For this review, take the finished solid that the model builds, in its own axes (mm). Face numbers are marked on the shaded views. A direction names the side the tool comes from. Give positions to 0.01 mm unless a question says otherwise; leave off trailing zeros. Order: outer loops, then holes, each group sorted by start corner. A loop starts at its lowest first (then second) coordinate and runs counter-clockwise, first axis right, second up. Notation, with made-up numbers: (-10, -11) - (37, -11) arc R32 cw to (37, 21) - close; hole circle Ø11 at (59, 86). An arc over 180 degrees is marked (long way). Use a Markdown table: item, result. Add a question column.
1) We need section B-B on z = 56.5. Write out the cut boundary in (x, y).
2) Clearance check with flat-ended pins moving along their axes: P1, Ø4, axis at x = -2, z = 64.5, coming from the +Y side; P2, Ø2, axis at x = -7, z = 50, coming from the -Y side; P3, Ø10, axis at x = -8, z = 71, coming from the -Y side; P4, Ø6, axis at y = -15.5, z = 69, coming from the +X side. State where each tip first meets the part, or that it passes through.
3) Mouldability with a two-part tool opening along X and no side actions: class the marked faces 4, 5 and 6 as released by +X, released by -X, zero draft, split by the parting line, or undercut.
4) Wall thickness on L1, parallel to Y at x = -10.5, z = 71.5; L2, parallel to X at y = -3, z = 60.5; L3, parallel to Z at x = -31.5, y = 24.5: over which ranges is each line inside the solid? List them lowest first.
5) Machinability: for the marked faces 1, 2 and 3, which of the approach directions +Z, -Z, +X, -X, +Y, -Y give a long, thin tool a straight path to every point of the face, cutting with its end or side? Answer none if there is none.
6) We need section C-C on x = -7. Give the number of separate pieces and of enclosed holes in the cut face, then the cut area to 3 significant figures.
7) We need section D-D on y = -59. Write out the cut boundary in (x, z), then the cut area to 3 significant figures.
8) We need section A-A on y = 0. Write out the cut boundary in (x, z).
```python
from build123d import *

# Parameters (mm, degrees)
EXTRUDE_DEPTH           = 10
EXTRUDE_PLACEMENT_ANGLE = 90
CYLINDER004_R           = 38
CYLINDER004_DEPTH       = 30
CYLINDER003_R           = 4
CYLINDER003_DEPTH       = 140
CYLINDER005_R           = 20
CYLINDER005_DEPTH       = 10
CYLINDER_R              = 46
CYLINDER_DEPTH          = 60


with BuildPart() as extrude_body:
    # path2399 → Extrude (new body)
    with BuildSketch(Plane(origin=(8.682374, 337.01873, 81), x_dir=(0, 1, 0), z_dir=(0, 0, 1))):
        with BuildLine():
            add(Edge.make_bspline(
                [(-1.415579, 5.024931), (-1.938341, -2.484397)],
                knots=[0, 0, 7.527502, 7.527502], degree=1))
            add(Edge.make_bspline(
                [(-1.938341, -2.484397), (-1.938341, -2.484397), (-2.134903, -2.858259), (-2.273136, -3.334737)],
                knots=[0, 0, 0, 0, 1, 1, 1, 1], degree=3))
            add(Edge.make_bspline(
                [(-2.273136, -3.334737), (-2.411369, -3.811216), (-2.443203, -4.128926), (-2.371685, -4.540758)],
                knots=[0, 0, 0, 0, 1, 1, 1, 1], degree=3))
            add(Edge.make_bspline(
                [(-2.371685, -4.540758), (-2.300167, -4.952591), (-2.218933, -5.672599), (-1.772797, -6.040394)],
                knots=[0, 0, 0, 0, 1, 1, 1, 1], degree=3))
            add(Edge.make_bspline(
                [(-1.772797, -6.040394), (-1.326661, -6.40819), (-0.861351, -6.572675), (-0.583202, -6.662312)],
                knots=[0, 0, 0, 0, 1, 1, 1, 1], degree=3))
            add(Edge.make_bspline(
                [(-0.583202, -6.662312), (-0.305053, -6.751952), (0.507781, -6.731952), (0.709843, -6.630052)],
                knots=[0, 0, 0, 0, 1, 1, 1, 1], degree=3))
            add(Edge.make_bspline(
                [(0.709843, -6.630052), (0.911905, -6.52815), (1.481843, -6.245909), (1.726833, -5.892641)],
                knots=[0, 0, 0, 0, 1, 1, 1, 1], degree=3))
            add(Edge.make_bspline(
                [(1.726833, -5.892641), (1.971823, -5.539373), (2.340182, -5.059724), (2.384256, -4.759981)],
                knots=[0, 0, 0, 0, 1, 1, 1, 1], degree=3))
            add(Edge.make_bspline(
                [(2.384256, -4.759981), (2.42833, -4.460237), (2.223091, -3.691858), (2.158411, -3.465999)],
                knots=[0, 0, 0, 0, 1, 1, 1, 1], degree=3))
            add(Edge.make_bspline(
                [(2.158411, -3.465999), (2.093732, -3.240141), (1.863634, -2.929328), (1.863634, -2.929328)],
                knots=[0, 0, 0, 0, 1, 1, 1, 1], degree=3))
            add(Edge.make_bspline(
                [(1.863634, -2.929328), (1.423808, 5.709855)],
                knots=[0, 0, 8.650371, 8.650371], degree=1))
            add(Edge.make_bspline(
                [(1.423808, 5.709855), (1.423808, 5.709855), (1.246198, 6.226563), (0.794563, 6.495307)],
                knots=[0, 0, 0, 0, 1, 1, 1, 1], degree=3))
            add(Edge.make_bspline(
                [(0.794563, 6.495307), (0.342929, 6.764051), (-0.057622, 6.753041), (-0.37358, 6.666974)],
                knots=[0, 0, 0, 0, 1, 1, 1, 1], degree=3))
            add(Edge.make_bspline(
                [(-0.37358, 6.666974), (-0.689538, 6.580907), (-1.208145, 6.230265), (-1.306201, 5.897514)],
                knots=[0, 0, 0, 0, 1, 1, 1, 1], degree=3))
            add(Edge.make_bspline(
                [(-1.306201, 5.897514), (-1.404257, 5.564763), (-1.415579, 5.024931), (-1.415579, 5.024931)],
                knots=[0, 0, 0, 0, 1, 1, 1, 1], degree=3))
        make_face()
    extrude(amount=EXTRUDE_DEPTH)


with BuildPart() as extrude_body_1:
    # Extrude placement: moved
    add(extrude_body.part.moved(Location((-13, -4, 402))).rotate(Axis((-13, -4, 402), (-1, 0, 0)), EXTRUDE_PLACEMENT_ANGLE))


with BuildPart() as cylinder004:
    # Cylinder004 → Cylinder004 (new body)
    with BuildSketch(Plane.XY.offset(56)):
        Circle(CYLINDER004_R)
    extrude(amount=CYLINDER004_DEPTH)


with BuildPart() as cut:
    # Cylinder003 → Cylinder003 (new body)
    with BuildSketch(Plane(origin=(0, 70, 65), x_dir=(1, 0, 0), z_dir=(0, -1, 0))):
        Circle(CYLINDER003_R)
    extrude(amount=CYLINDER003_DEPTH)

    # Cut: cut Cylinder004
    add(cylinder004.part, mode=Mode.SUBTRACT)


with BuildPart() as cut001:
    # Cylinder005 → Cylinder005 (new body)
    with BuildSketch(Plane(origin=(0, 80, 65), x_dir=(1, 0, 0), z_dir=(0, -1, 0))):
        Circle(CYLINDER005_R)
    extrude(amount=CYLINDER005_DEPTH)

    # Fusion: union Cut
    add(cut.part)

    # Cut001: cut Extrude body
    add(extrude_body_1.part, mode=Mode.SUBTRACT)


with BuildPart() as cylinder:
    # Cylinder → Cylinder (new body)
    with BuildSketch(Plane.XY):
        Circle(CYLINDER_R)
    extrude(amount=CYLINDER_DEPTH)


with BuildPart() as fusion001:
    # Sketch → Revolve (revolve)
    with BuildSketch(Plane.XZ):
        Polygon((0, 1), (34, 1), (38, 70), (42.057971, 70), (38, 0), (0, 0), align=None)
    revolve(axis=Axis((0, 0, 0), (0, 0, 1)))

    # Cut002: cut Cylinder
    add(cylinder.part, mode=Mode.SUBTRACT)

    # Fusion001: union Cut001
    add(cut001.part)


solid = fusion001.part
```
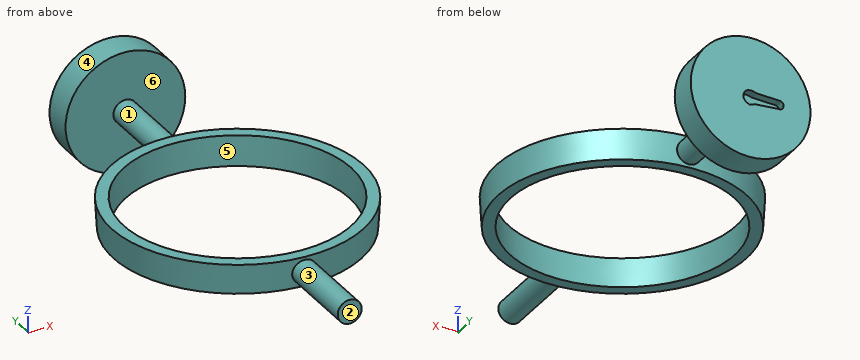
Checked values:
| question | item | result |
|---|---|---|
| 1 | outline | (-18.1, 70) - (18.1, 70) - (18.1, 80) - (-18.1, 80) - close |
| 2 | P1 | y = 80 |
| 2 | P2 | y = 70 |
| 2 | P3 | y = -41.94 |
| 2 | P4 | x = 40.11 |
| 3 | face 4 | split by the parting line |
| 3 | face 5 | undercut |
| 3 | face 6 | zero draft |
| 4 | L1 | 70 to 80 |
| 4 | L2 | -41.4 to -37.33, 37.33 to 41.4 |
| 4 | L3 | 60 to 70 |
| 5 | face 1 | none |
| 5 | face 2 | +Z, -Z, +X, -X, -Y |
| 5 | face 3 | -Y |
| 6 | separate pieces | 3 |
| 6 | enclosed holes | 0 |
| 6 | area | 448 mm² |
| 7 | outline | circle Ø8 at (0, 65) |
| 7 | area | 50.3 mm² |
| 8 | outline | (-42.06, 70) - (-41.48, 60) - (-37.42, 60) - (-38, 70) - close; (37.42, 60) - (41.48, 60) - (42.06, 70) - (38, 70) - close |
